Autodesk Inventor part; units mm, degrees
ref_plane "Work Plane2" through (127.5845, 533.2498, -119.0625) normal (0, 0, 1) x (1, 0, 0)
ref_plane "Work Plane3" through (116.586, 539.5998, -127) normal (0, 0, -1) x (-1, 0, 0)
ref_plane "YZ Plane" through (0, 0, 0) normal (1, 0, 0) x (0, 1, 0)
sketch "Sketch1" plane through (0, 0, 0) normal (0, 0, 1) x (1, 0, 0)
  line L0 (25.4, 0) -> (25.4, 359.664)
  line L1 (0, 359.664) -> (0, 0)
  arc A0 (0, 0) -> (25.4, 0) centre (12.7, 0) ccw
  arc A1 (25.4, 359.664) -> (0, 359.664) centre (12.7, 359.664) ccw
sketch "Sketch2" plane through (0, 0, 0) normal (0, 0, 1) x (1, 0, 0)
  line L0 (-287.7794, 186.1816) -> (71.8846, 186.1816) construction
  arc A0 (25.4, 359.664) -> (0, 359.664) centre (12.7, 359.664) ccw
  arc A1 (18.9244, 348.5939) -> (19.1748, 348.7385) centre (12.7, 359.664) ccw
  arc A2 (6.4756, 370.7341) -> (6.2252, 370.5895) centre (12.7, 359.664) ccw
  line L1 (12.7, 359.664) -> (220.472, 359.664) construction
  line L2 (23.6985, 353.314) -> (127.5845, 533.2498)
  line L3 (105.5875, 545.9498) -> (1.7015, 366.014)
  arc A3 (1.7015, 366.014) -> (23.6985, 353.314) centre (12.7, 359.664) ccw
  arc A4 (127.5845, 533.2498) -> (105.5875, 545.9498) centre (116.586, 539.5998) ccw
  point P0 (0, 0)
extrude "Extrusion1" add sketch "Sketch2" along normal blind 3.175
extrude "Extrusion2" add sketch "Sketch1" against normal blind 3.175
sketch "Sketch3" plane through (0, 0, 3.175) normal (0, 0, 1) x (1, 0, 0)
  circle A0 centre (12.7, 359.664) radius 2.5797
  point P0 (0, 0)
  dimension "d12" = 5.1594
extrude "Extrusion3" add sketch "Sketch3" along normal blind 3.175
sketch "Sketch4" plane through (0, 0, 0) normal (0, 0, -1) x (-1, 0, 0)
  arc A0 (-105.5875, 545.9498) -> (-127.5845, 533.2498) centre (-116.586, 539.5998) ccw
  circle A1 centre (-116.586, 539.5998) radius 12.7
  point P0 (0, 0)
extrude "Extrusion4" add sketch "Sketch4" along normal blind 127
ref_plane "Work Plane2" through (127.5845, 533.2498, -119.0625) normal (0, 0, 1) x (1, 0, 0)
ref_plane "Work Plane1" through (127.5845, 533.2498, 1.5875) normal (0, 0, 1) x (1, 0, 0)
ref_plane "Work Plane3" through (116.586, 539.5998, -127) normal (0, 0, -1) x (-1, 0, 0)
mirror "Mirror2" about plane through (116.586, 539.5998, -127) normal (0, 0, -1) of "Extrusion1", "Extrusion2"
sketch "Sketch5" plane through (116.586, 539.5998, -127) normal (0, 0, -1) x (-1, 0, 0)
  circle A0 centre (0, 0) radius 12.7
  circle A1 centre (0, 0) radius 12.7
  point P0 (116.586, -539.5998)
extrude "Extrusion5" add sketch "Sketch5" along normal blind 127
properties part number "cart handle"
Check sheet for the modelled part. Datum: model origin and axes. Units: mm. A direction names the side the tool comes from. Round coordinates to 2 decimals unless told otherwise and drop trailing zeros. Order: outer loops, then holes, each group sorted by start corner. A loop starts at its lowest first (then second) coordinate and runs counter-clockwise, first axis right, second up. Notation, with made-up numbers: (0.25, 14) -> (10.25, 14) arc R18 cw to (10.25, 18) -> close; hole circle Ø1 at (48.25, 69). An arc over 180 degrees is marked (long way). One line per item, written item: value. Start each with the question number.
Q1. Mould release check, pull along Z, two halves, no side actions. Record for faces 1 (the face through (105.848, 532.819, -153.444)), 2 (the face through (64, 450, 3.175)), 3 (the face through (123.176, 550.456, -255.565)): pulls with the +Z half, pulls with the -Z half, needs draft (parallel to the pull), parting line crosses it, or undercut.
Q2. Cross-section at A-A (x = 46). Record the boundary of the cut face in (y, z) (3 decimals).
Q3. Gauge pin test, flat ends, axial feed: pin 1 Ø20.5 at (x, y) = (11, 232) entering from -Z; pin 2 Ø20.5 at (x, y) = (8.5, 90.5) entering from +Z; pin 3 Ø1 at (x, z) = (110, -32) entering from -Y. Record the tip position at first contact, or that the pin passes through.
Q4. Set-up check for faces 4 (the face through (6.45, 348.61, 1.57)), 5 (the face through (13, 183, -250.825)), 6 (the face through (8.1, 371.5, -252.6)), 7 (the face through (6.128, 348.796, -255.565)), 8 (the face through (12.979, -12.697, -252.435)): record each of +Z, -Z, +X, -X, +Y, -Y from which the full face is reachable in a straight line by a thin tool's end or side.
Q5. Thickness scan on line 1 (Y direction, x = 114, z = -145). Record the ranges inside material, lowest first.
Q6. Cross-section at B-B (z = -62.5). Record the boundary of the cut face in (x, y), and give its area (3 significant figures).
Completed:
1. face 1: undercut
1. face 2: pulls with the +Z half
1. face 3: needs draft
2. outline: (391.941, -257.175) -> (442.741, -257.175) -> (442.741, -254) -> (391.941, -254) -> close; (391.941, 0) -> (442.741, 0) -> (442.741, 3.175) -> (391.941, 3.175) -> close
3. pin 1: stops at z = -254
3. pin 2: stops at z = 0
3. pin 3: stops at y = 528.45
4. face 4: +Z, -Y
4. face 5: +X, -X, +Y, -Y
4. face 6: +Y
4. face 7: -Z, -Y
4. face 8: +Z, -Z, -Y
5. line 1: y = 527.17 to 552.03
6. outline: circle Ø25.4 at (116.59, 539.6)
6. area: 507 mm²
